Part model, mm, in its own coordinate system. A direction names the side the tool comes from. Round coordinates to 2 decimals unless told otherwise and drop trailing zeros. Loops run counter-clockwise (first coordinate to the right, second up) from the corner with the lowest first, then second, coordinate; pieces in that order, holes last. Notation, with made-up numbers: M -7,-15.5 L 25,-15.5 A13 ccw 25,-10.5 Z; hole C -37.5,84 d1. An arc over 180 degrees is marked long. Write each question's results on one line, items separated by ' | '.
from build123d import *

# Parameters (mm, degrees)
SKETCH1_R                = 2
BOSS_EXTRUDE1_DEPTH      = 2.5
BOSS_EXTRUDE2_DEPTH      = 24.645
BOSS_EXTRUDE2_DEPTH_BACK = 24.645
SKETCH4_W                = 49.29
SKETCH4_H                = 2.5
BOSS_EXTRUDE4_DEPTH      = 14
BOSS_EXTRUDE6_DEPTH      = 1.5
BOSS_EXTRUDE7_START      = 12.5
BOSS_EXTRUDE7_DEPTH      = 1.5
BOSS_EXTRUDE8_START      = 1.5
BOSS_EXTRUDE8_DEPTH      = 1.5
BOSS_EXTRUDE9_START      = 11
BOSS_EXTRUDE9_DEPTH      = 1.5
BOSS_EXTRUDE10_START     = 6.5
BOSS_EXTRUDE10_DEPTH     = 3
BOSS_EXTRUDE11_START     = 20
BOSS_EXTRUDE11_DEPTH     = 3


with BuildPart() as part:
    # Sketch1 → Boss-Extrude1 (new body)
    with BuildSketch(Plane(origin=(0, 0, 0), x_dir=(1, 0, 0), z_dir=(0, 1, 0))):
        Polygon((-29.841152423, 0), (-24.645, 9), (24.645, 9), (29.841152423, 0), align=None)
        with Locations(Location((-14.92, 4.5, 0), (0, 0, 270))):
            Circle(SKETCH1_R, mode=Mode.SUBTRACT)
        with Locations(Location((14.92, 4.5, 0), (0, 0, 270))):
            Circle(SKETCH1_R, mode=Mode.SUBTRACT)
    extrude(amount=BOSS_EXTRUDE1_DEPTH)

    # Sketch3 → Boss-Extrude2 (add, two sides: drawn at the far end of the back side and taken through both)
    with BuildSketch(Plane(origin=(0, 0, 0), x_dir=(0, 0, -1), z_dir=(1, 0, 0)).offset(-BOSS_EXTRUDE2_DEPTH_BACK)):
        with BuildLine():
            Line((9, 0), (9, 2.5))
            ThreePointArc((9, 2.5), (11.121320344, 3.378679656), (12, 5.5))
            Line((12, 5.5), (14.5, 5.5))
            ThreePointArc((14.5, 5.5), (12.889087297, 1.610912703), (9, 0))
        make_face()
    extrude(amount=BOSS_EXTRUDE2_DEPTH + BOSS_EXTRUDE2_DEPTH_BACK)

    # Sketch4 → Boss-Extrude4 (add)
    with BuildSketch(Plane(origin=(0, 5.5, 0), x_dir=(1, 0, 0), z_dir=(0, 1, 0))):
        with BuildLine():
            Line((-49.558586772, 12), (-24.645, 12))
            Line((-24.645, 12), (-24.645, 14.5))
            Line((-24.645, 14.5), (-44.793833293, 14.5))
            ThreePointArc((-44.793833293, 14.5), (-67.270294591, 10.832042119), (-87.5, 0.372393629))
            Line((-87.5, 0.372393629), (-87.5, -2.532989082))
            ThreePointArc((-87.5, -2.532989082), (-69.603961511, 7.539151784), (-49.558586772, 12))
        make_face()
        with Locations((0, 13.25)):
            Rectangle(SKETCH4_W, SKETCH4_H)
        with BuildLine():
            Line((24.645, 12), (44.795929756, 12))
            ThreePointArc((44.795929756, 12), (67.371893328, 8.158628084), (87.5, -2.763349356))
            Line((87.5, -2.763349356), (87.5, 0.372340835))
            ThreePointArc((87.5, 0.372340835), (67.265225258, 10.833674125), (44.783151118, 14.5))
            Line((44.783151118, 14.5), (24.645, 14.5))
            Line((24.645, 14.5), (24.645, 12))
        make_face()
    extrude(amount=BOSS_EXTRUDE4_DEPTH)

    # Sketch4<4> → Boss-Extrude6 (add)
    with BuildSketch(Plane(origin=(0, 5.5, 0), x_dir=(1, 0, 0), z_dir=(0, 1, 0))):
        with BuildLine():
            ThreePointArc((44.783151118, 14.5), (67.265225258, 10.833674125), (87.5, 0.372340835))
            Line((87.5, 0.372340835), (87.5, 3.872340835))
            ThreePointArc((87.5, 3.872340835), (67.030937137, 13.899537079), (44.500036985, 17.347106846))
            Line((44.500036985, 17.347106846), (-44.499963015, 17.347150533))
            ThreePointArc((-44.499963015, 17.347150533), (-67.030900409, 13.89959402), (-87.5, 3.872393629))
            Line((-87.5, 3.872393629), (-87.5, 0.372393629))
            ThreePointArc((-87.5, 0.372393629), (-67.270294591, 10.832042119), (-44.793833293, 14.5))
            Line((-44.793833293, 14.5), (-24.645, 14.5))
            Line((-24.645, 14.5), (24.645, 14.5))
            Line((24.645, 14.5), (44.783151118, 14.5))
        make_face()
        with BuildLine():
            ThreePointArc((87.5, 3.872340835), (67.030937113, 13.899537086), (44.500036985, 17.347106846))
            Line((44.500036985, 17.347106846), (-44.499963015, 17.347150533))
            ThreePointArc((-44.499963015, 17.347150533), (-67.030900409, 13.89959402), (-87.5, 3.872393629))
            Line((-87.5, 3.872393629), (-87.5, 5.372393629))
            ThreePointArc((-87.5, 5.372393629), (-66.991859053, 15.206396924), (-44.499962408, 18.583681514))
            Line((-44.499962408, 18.583681514), (44.500037592, 18.583637828))
            ThreePointArc((44.500037592, 18.583637828), (66.991896325, 15.206339771), (87.5, 5.372340835))
            Line((87.5, 5.372340835), (87.5, 3.872340835))
        make_face()
    extrude(amount=BOSS_EXTRUDE6_DEPTH)

    # Sketch4<5> → Boss-Extrude7 (add)
    with BuildSketch(Plane(origin=(0, 5.5, 0), x_dir=(1, 0, 0), z_dir=(0, 1, 0)).offset(BOSS_EXTRUDE7_START)):
        with BuildLine():
            ThreePointArc((44.783151118, 14.5), (67.265225258, 10.833674125), (87.5, 0.372340835))
            Line((87.5, 0.372340835), (87.5, 3.872340835))
            ThreePointArc((87.5, 3.872340835), (67.030937137, 13.899537079), (44.500036985, 17.347106846))
            Line((44.500036985, 17.347106846), (-44.499963015, 17.347150533))
            ThreePointArc((-44.499963015, 17.347150533), (-67.030900409, 13.89959402), (-87.5, 3.872393629))
            Line((-87.5, 3.872393629), (-87.5, 0.372393629))
            ThreePointArc((-87.5, 0.372393629), (-67.270294591, 10.832042119), (-44.793833293, 14.5))
            Line((-44.793833293, 14.5), (-24.645, 14.5))
            Line((-24.645, 14.5), (24.645, 14.5))
            Line((24.645, 14.5), (44.783151118, 14.5))
        make_face()
        with BuildLine():
            ThreePointArc((87.5, 3.872340835), (67.030937113, 13.899537086), (44.500036985, 17.347106846))
            Line((44.500036985, 17.347106846), (-44.499963015, 17.347150533))
            ThreePointArc((-44.499963015, 17.347150533), (-67.030900409, 13.89959402), (-87.5, 3.872393629))
            Line((-87.5, 3.872393629), (-87.5, 5.372393629))
            ThreePointArc((-87.5, 5.372393629), (-66.991859053, 15.206396924), (-44.499962408, 18.583681514))
            Line((-44.499962408, 18.583681514), (44.500037592, 18.583637828))
            ThreePointArc((44.500037592, 18.583637828), (66.991896325, 15.206339771), (87.5, 5.372340835))
            Line((87.5, 5.372340835), (87.5, 3.872340835))
        make_face()
    extrude(amount=BOSS_EXTRUDE7_DEPTH)

    # Sketch4<6> → Boss-Extrude8 (add)
    with BuildSketch(Plane(origin=(0, 5.5, 0), x_dir=(1, 0, 0), z_dir=(0, 1, 0)).offset(BOSS_EXTRUDE8_START)):
        with BuildLine():
            ThreePointArc((87.5, 3.872340835), (67.030937113, 13.899537086), (44.500036985, 17.347106846))
            Line((44.500036985, 17.347106846), (-44.499963015, 17.347150533))
            ThreePointArc((-44.499963015, 17.347150533), (-67.030900409, 13.89959402), (-87.5, 3.872393629))
            Line((-87.5, 3.872393629), (-87.5, 5.372393629))
            ThreePointArc((-87.5, 5.372393629), (-66.991859053, 15.206396924), (-44.499962408, 18.583681514))
            Line((-44.499962408, 18.583681514), (44.500037592, 18.583637828))
            ThreePointArc((44.500037592, 18.583637828), (66.991896325, 15.206339771), (87.5, 5.372340835))
            Line((87.5, 5.372340835), (87.5, 3.872340835))
        make_face()
    extrude(amount=BOSS_EXTRUDE8_DEPTH)

    # Sketch4<8> → Boss-Extrude9 (add)
    with BuildSketch(Plane(origin=(0, 5.5, 0), x_dir=(1, 0, 0), z_dir=(0, 1, 0)).offset(BOSS_EXTRUDE9_START)):
        with BuildLine():
            ThreePointArc((87.5, 3.872340835), (67.030937113, 13.899537086), (44.500036985, 17.347106846))
            Line((44.500036985, 17.347106846), (-44.499963015, 17.347150533))
            ThreePointArc((-44.499963015, 17.347150533), (-67.030900409, 13.89959402), (-87.5, 3.872393629))
            Line((-87.5, 3.872393629), (-87.5, 5.372393629))
            ThreePointArc((-87.5, 5.372393629), (-66.991859053, 15.206396924), (-44.499962408, 18.583681514))
            Line((-44.499962408, 18.583681514), (44.500037592, 18.583637828))
            ThreePointArc((44.500037592, 18.583637828), (66.991896325, 15.206339771), (87.5, 5.372340835))
            Line((87.5, 5.372340835), (87.5, 3.872340835))
        make_face()
    extrude(amount=BOSS_EXTRUDE9_DEPTH)

    # Sketch5 → Boss-Extrude10 (add)
    with BuildSketch(Plane(origin=(0, 0, 0), x_dir=(0, 0, -1), z_dir=(1, 0, 0)).offset(BOSS_EXTRUDE10_START)):
        with BuildLine():
            Line((11.977989331, 19.5), (0, 2.5))
            Line((0, 2.5), (9, 2.5))
            ThreePointArc((9, 2.5), (11.113552723, 3.380024256), (11.977989331, 5.5))
            Line((11.977989331, 5.5), (11.977989331, 19.5))
        make_face()
    boss_extrude10 = extrude(amount=BOSS_EXTRUDE10_DEPTH)

    # Sketch5<3> → Boss-Extrude11 (add)
    with BuildSketch(Plane(origin=(0, 0, 0), x_dir=(0, 0, -1), z_dir=(1, 0, 0)).offset(BOSS_EXTRUDE11_START)):
        with BuildLine():
            Line((11.977989331, 19.5), (0, 2.5))
            Line((0, 2.5), (9, 2.5))
            ThreePointArc((9, 2.5), (11.113552723, 3.380024256), (11.977989331, 5.5))
            Line((11.977989331, 5.5), (11.977989331, 19.5))
        make_face()
    boss_extrude11 = extrude(amount=BOSS_EXTRUDE11_DEPTH)

    # Mirror1: Boss-Extrude10, Boss-Extrude11 across plane
    add(boss_extrude10.mirror(Plane(origin=(0, 0, 0), x_dir=(0, 0, 1), z_dir=(1, 0, 0))))
    add(boss_extrude11.mirror(Plane(origin=(0, 0, 0), x_dir=(0, 0, 1), z_dir=(1, 0, 0))))


solid = part.part
Item 1: Band-saw the part on B-B on y = 14.5. Give the cut face in (x, z), and give its area (3 significant figures).
Filled sheet:
outline: M -87.5,-0.37 A72.5 ccw -44.79,-14.5 L 44.78,-14.5 A72.5 ccw 87.5,-0.37 L 87.5,2.76 A70 cw 44.8,-12 L -49.56,-12 A70.18 cw -87.5,2.53 Z; M -23,-11.98 L -20,-11.98 L -20,-8.46 L -23,-8.46 Z; M -9.5,-11.98 L -6.5,-11.98 L -6.5,-8.46 L -9.5,-8.46 Z; M 6.5,-11.98 L 9.5,-11.98 L 9.5,-8.46 L 6.5,-8.46 Z; M 20,-11.98 L 23,-11.98 L 23,-8.46 L 20,-8.46 Z | area: 488 mm^2
Item 2: Band-saw the part on A-A on x = 14.92. Give the cut face in (y, z).
Filled sheet:
outline: M 0,-9 A5.5 ccw 5.5,-14.5 L 5.5,-18.58 L 8.5,-18.58 L 8.5,-17.35 L 7,-17.35 L 7,-14.5 L 18,-14.5 L 18,-17.35 L 16.5,-17.35 L 16.5,-18.58 L 19.5,-18.58 L 19.5,-12 L 5.5,-12 A3 cw 2.5,-9 L 2.5,-6.5 L 0,-6.5 Z; M 0,-2.5 L 2.5,-2.5 L 2.5,0 L 0,0 Z
Item 3: Which spindle directions (+Z, -Z, +X, -X, +Y, -Y) get a long thin tool onto all of the face, cutting with end or side? Do faces 4 (the cylindrical face through (67.067, 12.402, -8.263)), 5 (the flat face through (6.5, 7, -9)), 6 (the flat face through (-24.645, 3, -12)), 7 (the cylindrical face through (67.34, 17.24, -13.8)). Say none if no direction does.
Filled sheet:
face 4: +Z, +Y, -Y | face 5: +Z, +Y | face 6: -Z, -X, -Y | face 7: none
Item 4: Two-plate mould, pull along Z, no slides. Class faces 1 (the flat face through (0, 7, -15)), 2 (the cylindrical face through (-67.3, 17.98, -15.11)), 3 (the flat face through (20, 7, -9)): +Z half, -Z half, draft (parallel to the pull), parting line (faces both ways), or undercut.
Filled sheet:
face 1: undercut | face 2: -Z half | face 3: draft
Item 5: Drop flat-ended pins along their axis: P1, Ø3.5, axis at x = -25.5, z = -5, coming from the +Y side; P2, Ø1, axis at x = -55, y = 15.5, coming from the -Z side; P3, Ø1.6, axis at x = -18.5, y = 8, coming from the +Z side. Give the stop position or say it passes through.
Filled sheet:
P1: y = 2.5 | P2: z = -13.81 | P3: z = -12
Item 6: Band-saw the part on D-D on x = 51.5. Give the cut face in (y, z).
Filled sheet:
outline: M 5.5,-18.26 L 8.5,-18.26 L 8.5,-17.02 L 7,-17.02 L 7,-14.16 L 18,-14.16 L 18,-17.02 L 16.5,-17.02 L 16.5,-18.26 L 19.5,-18.26 L 19.5,-11.65 L 5.5,-11.65 Z
Item 7: Band-saw the part on C-C on x = 34. Give the cut face in (y, z).
Filled sheet:
outline: M 5.5,-18.58 L 8.5,-18.58 L 8.5,-17.35 L 7,-17.35 L 7,-14.5 L 18,-14.5 L 18,-17.35 L 16.5,-17.35 L 16.5,-18.58 L 19.5,-18.58 L 19.5,-12 L 5.5,-12 Z
Item 8: Wall check: L1, parallel to X at y = 2.75, z = -0.25; L2, parallel to Y at x = 9, z = -17; L3, parallel to X at y = 0.6, z = -4.5. Give the ranges that are in metal, low to high.
Filled sheet:
L1: -23 to -20, -9.5 to -6.5, 6.5 to 9.5, 20 to 23 | L2: 5.5 to 7, 18 to 19.5 | L3: -27.24 to -16.92, -12.92 to 12.92, 16.92 to 27.24
